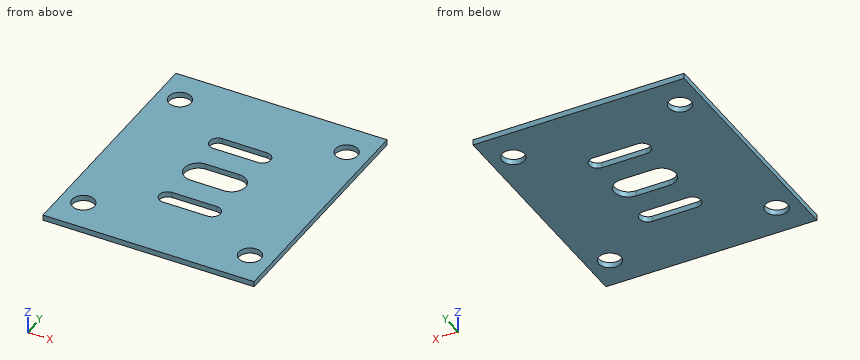
```python
from build123d import *

# Parameters (mm, degrees)
SKETCH1_W               = 38
SKETCH1_H               = 44
SKETCH1_R               = 2
BOSS_EXTRUDE1_DEPTH     = 1
CUT_EXTRUDE1_DEPTH      = 30.086079144
CUT_EXTRUDE1_DEPTH_BACK = 30.086079144


with BuildPart() as part:
    # Sketch1 → Boss-Extrude1 (new body)
    with BuildSketch(Plane.XY):
        Rectangle(SKETCH1_W, SKETCH1_H)
        with Locations((-15, 16)):
            Circle(SKETCH1_R, mode=Mode.SUBTRACT)
        with Locations(Location((-15, -16, 0), (0, 0, 180))):
            Circle(SKETCH1_R, mode=Mode.SUBTRACT)
        with Locations((15, -16)):
            Circle(SKETCH1_R, mode=Mode.SUBTRACT)
        with Locations(Location((15, 16, 0), (0, 0, 180))):
            Circle(SKETCH1_R, mode=Mode.SUBTRACT)
    extrude(amount=BOSS_EXTRUDE1_DEPTH)

    # Sketch2 → Cut-Extrude1 (cut, two sides: drawn at the far end of the back side and taken through both)
    with BuildSketch(Plane.XY.offset(-CUT_EXTRUDE1_DEPTH_BACK)):
        with BuildLine():
            Line((-3, 2.5), (3, 2.5))
            ThreePointArc((3, 2.5), (5.5, 0), (3, -2.5))
            Line((3, -2.5), (-3, -2.5))
            ThreePointArc((-3, -2.5), (-5.5, 0), (-3, 2.5))
        make_face()
        with BuildLine():
            Line((-4, 9.827019403), (4, 9.827019403))
            ThreePointArc((4, 9.827019403), (5.5, 8.327019403), (4, 6.827019403))
            Line((4, 6.827019403), (-4, 6.827019403))
            ThreePointArc((-4, 6.827019403), (-5.5, 8.327019403), (-4, 9.827019403))
        make_face()
        with BuildLine():
            Line((-4, -9.827019403), (4, -9.827019403))
            ThreePointArc((4, -9.827019403), (5.5, -8.327019403), (4, -6.827019403))
            Line((4, -6.827019403), (-4, -6.827019403))
            ThreePointArc((-4, -6.827019403), (-5.5, -8.327019403), (-4, -9.827019403))
        make_face()
    extrude(amount=CUT_EXTRUDE1_DEPTH + CUT_EXTRUDE1_DEPTH_BACK, mode=Mode.SUBTRACT)


solid = part.part
```
The model under review builds one solid part; all positions refer to its coordinate system, in mm. Round coordinates to 2 decimals unless told otherwise and drop trailing zeros. Loops run counter-clockwise (first coordinate to the right, second up) from the corner with the lowest first, then second, coordinate; pieces in that order, holes last.
1) Clearance check with flat-ended pins moving along their axes: P1, Ø8, axis at x = -8, y = 4.5, coming from the -Z side; P2, Ø2.5, axis at x = 15, y = -16, coming from the -Z side. State where each tip first meets the part, or that it passes through.
Values follow:
P1: stops at z = 0
P2: passes through
2) Consider section C-C on z = 0.65. State the section outline as (x, y) points, then the cut area to 3 significant figures.
Values follow:
outline: (-19, -22) - (19, -22) - (19, 22) - (-19, 22) - close; hole circle Ø4 at (-15, -16); hole circle Ø4 at (-15, 16); hole (-4, -9.83) - (4, -9.83) arc R1.5 ccw to (4, -6.83) - (-4, -6.83) arc R1.5 ccw to start; hole (-4, 6.83) - (4, 6.83) arc R1.5 ccw to (4, 9.83) - (-4, 9.83) arc R1.5 ccw to start; hole (-3, -2.5) - (3, -2.5) arc R2.5 ccw to (3, 2.5) - (-3, 2.5) arc R2.5 ccw to start; hole circle Ø4 at (15, -16); hole circle Ø4 at (15, 16)
area: 1,510 mm2
3) Consider section A-A on y = 8.5. State the section outline as (x, z) points.
Values follow:
outline: (-19, 0) - (-5.49, 0) - (-5.49, 1) - (-19, 1) - close; (5.49, 0) - (19, 0) - (19, 1) - (5.49, 1) - close
4) Consider section B-B on x = 15. State the section outline as (y, z) points, then the cut area to 3 significant figures.
Values follow:
outline: (-22, 0) - (-18, 0) - (-18, 1) - (-22, 1) - close; (-14, 0) - (14, 0) - (14, 1) - (-14, 1) - close; (18, 0) - (22, 0) - (22, 1) - (18, 1) - close
area: 36.0 mm2
5) Consider section D-D on y = -16. State the section outline as (x, z) points, then the cut area to 3 significant figures.
Values follow:
outline: (-19, 0) - (-17, 0) - (-17, 1) - (-19, 1) - close; (-13, 0) - (13, 0) - (13, 1) - (-13, 1) - close; (17, 0) - (19, 0) - (19, 1) - (17, 1) - close
area: 30.0 mm2
6) Wall thickness on line 1 along Y through (x, z) = (15, 0.3); line 2 along Y through (x, z) = (-4, 0.25); line 3 along Y through (x, z) = (-3.5, 0.5): over which ranges is each line inside the solid? List them lowest first.
Values follow:
line 1: y = -22 to -18, -14 to 14, 18 to 22
line 2: y = -22 to -9.83, -6.83 to -2.29, 2.29 to 6.83, 9.83 to 22
line 3: y = -22 to -9.83, -6.83 to -2.45, 2.45 to 6.83, 9.83 to 22
